```python
from build123d import *

# Parameters (mm, degrees)
SKETCH_2_R          = 6.56
SKETCH_1_R          = 18.55
SKETCH_3_R          = 30
EXTRUDE_2_DEPTH     = 10
SKETCH_3_5_R        = 30
CUT_EXTRUDE_2_DEPTH = 10
SKETCH_4_R          = 3
CUT_EXTRUDE_3_DEPTH = 22


with BuildPart() as part:
    # 스케치2 → 로프트1 section 0
    with BuildSketch(Plane(origin=(0, 56.41, 0), x_dir=(1, 0, 0), z_dir=(0, 1, 0))):
        Circle(SKETCH_2_R)
    # 스케치1 → 로프트1 section 1
    with BuildSketch(Plane(origin=(0, 0, 0), x_dir=(1, 0, 0), z_dir=(0, 1, 0))):
        Circle(SKETCH_1_R)
    loft()

    # 스케치3 → 보스-돌출2 (add)
    with BuildSketch(Plane(origin=(0, 0, 0), x_dir=(1, 0, 0), z_dir=(0, 1, 0))):
        with Locations(Location((0, 0, 0), (0, 0, 270))):
            Circle(SKETCH_3_R)
    extrude(amount=-EXTRUDE_2_DEPTH)

    # 스케치3<5> → 컷-돌출2 (cut)
    with BuildSketch(Plane(origin=(0, 0, 0), x_dir=(1, 0, 0), z_dir=(0, 1, 0))):
        with Locations((30, 0)):
            Circle(SKETCH_3_5_R)
    extrude(amount=-CUT_EXTRUDE_2_DEPTH, mode=Mode.SUBTRACT)

    # 스케치4 → 컷-돌출3 (cut)
    with BuildSketch(Plane(origin=(0, 56.41, 0), x_dir=(1, 0, 0), z_dir=(0, 1, 0))):
        with Locations(Location((0, 0, 0), (0, 0, 270))):
            Circle(SKETCH_4_R)
    extrude(amount=-CUT_EXTRUDE_3_DEPTH, mode=Mode.SUBTRACT)


solid = part.part
```
Can you work these out from the model? Positions are in its coordinate system, mm. A direction names the side the tool comes from. Coordinates: 2 decimals unless noted, no trailing zeros. Loops run counter-clockwise (first coordinate to the right, second up) from the corner with the lowest first, then second, coordinate; pieces in that order, holes last. Notation, with made-up numbers: M -27.75,-0.5 L 13.25,-0.5 A32 cw 13.25,30.5 Z; hole C 38.25,-33 d9. An arc over 180 degrees is marked long. Put each result on its own line as item: value. Start each with the question number.
(1) Imagine slicing it at B-B on x = -26. List the corners of the cut face in (y, z) for me, and give its area (3 significant figures).
(2) Will these pins go through, and if not, where does the flat tip stop? pin 1 Ø4 at (y, z) = (14.5, -11.5) entering from +X; pin 2 Ø20.5 at (x, z) = (5, 6.5) entering from -Y; pin 3 Ø5 at (x, y) = (-18.5, 23) entering from -Z; pin 4 Ø1 at (x, y) = (6.5, 14.5) entering from -Z.
(3) I need wall thicknesses on probe 1 along Y at (x, z) = (4.5, -19); probe 2 along X at (y, z) = (39.5, 0); probe 3 along X at (y, z) = (48, 0). Which ranges of each line are inside material? Lowest first, please.
(4) Which directions (+Z, -Z, +X, -X, +Y, -Y) give clear straight access to the entire face, cutting with the end or side of a thin tool? Please do faces 4 (the face through (0, 34.41, 0)), 5 (the face through (1, 56.41, 3)), 6 (the face through (9, 0, 0)).
(5) Imagine slicing it at A-A on y = 52.5. List the corners of the cut face in (x, z) for me, and give its area (3 significant figures).
(6) Imagine slicing it at C-C on y = 5.5. List the corners of the cut face in (x, z) for me, and give its area (3 significant figures).
(7) We'd pull the mould along Z, two halves only. Please class faces 1 (the face through (-29.987, -4.93, -0.88)), 2 (the face through (-7, -10, 0)), 3 (the face through (0.9, 45.56, 2.86)): +Z half, -Z half, draft (parallel to the pull), parting line (faces both ways), or undercut.
Worked answers:
1. outline: M -10,-14.97 L 0,-14.97 L 0,14.97 L -10,14.97 Z
1. area: 299 mm2
2. pin 1: stops at x = 12.3
2. pin 2: stops at y = -10
2. pin 3: passes through
2. pin 4: stops at z = -14.29
3. probe 1: y = -10 to 0
3. probe 2: x = -10.15 to -3, 3 to 10.15
3. probe 3: x = -8.35 to -3, 3 to 8.35
4. face 4: +Y
4. face 5: +Z, -Z, +X, -X, +Y
4. face 6: +X, -Y
5. outline: C 0,0 d14.78; hole C 0,0 d6
5. area: 143 mm2
6. outline: C 0,0 d34.76
6. area: 949 mm2
7. face 1: parting line
7. face 2: draft
7. face 3: undercut
